```python
from build123d import *

# Parameters (mm, degrees)
SKETCH1_R                                         = 2.5
BOSS_EXTRUDE1_DEPTH                               = 5
SKETCH2_W                                         = 5
SKETCH2_H                                         = 55
BOSS_EXTRUDE2_DEPTH                               = 25
SKETCH3_W                                         = 72.3
SKETCH3_H                                         = 55
BOSS_EXTRUDE3_DEPTH                               = 5
BOSS_EXTRUDE4_DEPTH                               = 5
CUT_EXTRUDE1_REACH                                = 7
SKETCH5_R                                         = 2.5
CSK_FOR_M2_5_FLAT_HEAD_MACHINE_SCREW1_D           = 2.9
CSK_FOR_M2_5_FLAT_HEAD_MACHINE_SCREW1_CSINK_D     = 5.5
CSK_FOR_M2_5_FLAT_HEAD_MACHINE_SCREW1_CSINK_ANGLE = 90


with BuildPart() as part:
    # Sketch1 → Boss-Extrude1 (new body)
    with BuildSketch(Plane(origin=(0, 0, 0), x_dir=(0, 0, -1), z_dir=(1, 0, 0))):
        Polygon((-27.5, 17.5), (-17.5, 27.5), (17.5, 27.5), (27.5, 17.5), (27.5, -27.5), (-27.5, -27.5), align=None)
        Circle(SKETCH1_R, mode=Mode.SUBTRACT)
    extrude(amount=BOSS_EXTRUDE1_DEPTH)

    # Sketch2 → Boss-Extrude2 (add)
    with BuildSketch(Plane.XZ.offset(27.5)):
        with Locations((2.5, 0)):
            Rectangle(SKETCH2_W, SKETCH2_H)
    extrude(amount=BOSS_EXTRUDE2_DEPTH)

    # Sketch3 → Boss-Extrude3 (add)
    with BuildSketch(Plane.XZ.offset(52.5)):
        with Locations((-36.15, 0)):
            Rectangle(SKETCH3_W, SKETCH3_H)
    extrude(amount=-BOSS_EXTRUDE3_DEPTH)

    # Sketch4 → Boss-Extrude4 (add)
    with BuildSketch(Plane.ZY.offset(72.3)):
        Polygon((-17.5, 27.5), (-27.5, 17.5), (-27.5, -47.5), (27.5, -47.5), (27.5, 17.5), (17.5, 27.5), align=None)
    extrude(amount=-BOSS_EXTRUDE4_DEPTH)

    # Sketch5 → Cut-Extrude1 (cut, up to next)
    with BuildSketch(Plane(origin=(-67.3, 0, 0), x_dir=(0, 0, -1), z_dir=(1, 0, 0)), mode=Mode.PRIVATE) as cut_extrude1_sk1:
        Circle(SKETCH5_R)
    cut_extrude1_tool1 = extrude(cut_extrude1_sk1.sketch, amount=-CUT_EXTRUDE1_REACH, mode=Mode.PRIVATE) & part.part
    add(cut_extrude1_tool1.solids().sort_by_distance((-67.3, 0, 0))[0], mode=Mode.SUBTRACT)

    # CSK for M2.5 Flat Head Machine Screw1 (through all)
    with Locations(Plane(origin=(0, -47.5, 0), x_dir=(1, 0, 0), z_dir=(0, 1, 0))):
        with Locations((-16.15, 15), (-16.15, -15), (-46.15, -15), (-46.15, 15)):
            CounterSinkHole(CSK_FOR_M2_5_FLAT_HEAD_MACHINE_SCREW1_D / 2, CSK_FOR_M2_5_FLAT_HEAD_MACHINE_SCREW1_CSINK_D / 2, counter_sink_angle=CSK_FOR_M2_5_FLAT_HEAD_MACHINE_SCREW1_CSINK_ANGLE)


solid = part.part
```
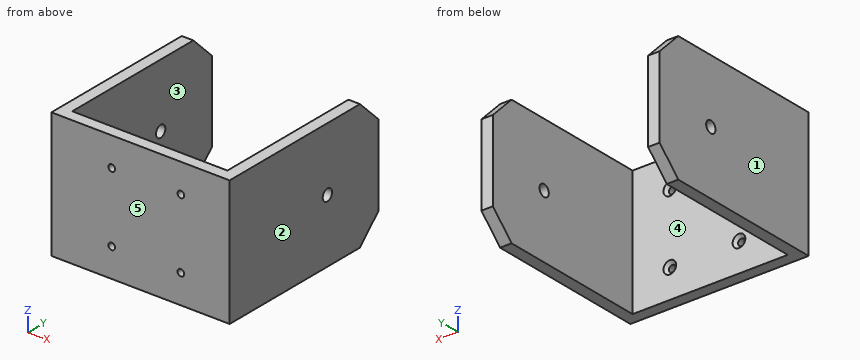
Input: part model. Units: mm. Frame: model coordinates. Face numbers are marked on the shaded views. A direction names the side the tool comes from. Coordinates: 2 decimals unless noted, no trailing zeros. Write each loop counter-clockwise with the first axis right and the second up, starting at its lowest first coordinate (ties: lowest second). Pieces come first, ordered by that corner, then holes. Notation, with made-up numbers: M -27.75,51.5 L -7.75,51.5 A26 cw -7.75,85.5 Z; hole C -1.5,32 d9. An arc over 180 degrees is marked long. Use one line per item in the form item = value.
Q1. Draft query along X for the marked faces 1, 2 and 3. Return one class per face: released by +X, released by -X, zero draft, split by the parting line, or undercut.
Answer below:
face_1 = released by -X
face_2 = released by +X
face_3 = undercut
Q2. Section D-D (y = -44). Return loops of the section in (x, z).
Answer below:
outline = M -72.3,-27.5 L -67.3,-27.5 L -67.3,27.5 L -72.3,27.5 Z; M 0,-27.5 L 5,-27.5 L 5,27.5 L 0,27.5 Z
Q3. Section B-B (y = 0). Return loops of the section in (x, z).
Answer below:
outline = M -72.3,-27.5 L -67.3,-27.5 L -67.3,-2.5 L -72.3,-2.5 Z; M -72.3,2.5 L -67.3,2.5 L -67.3,27.5 L -72.3,27.5 Z; M 0,-27.5 L 5,-27.5 L 5,-2.5 L 0,-2.5 Z; M 0,2.5 L 5,2.5 L 5,27.5 L 0,27.5 Z
Q4. Material intervals for probe 1 along X at (y, z) = (-50, -15); probe 2 along Z at (x, y) = (-46, -51); probe 3 along X at (y, z) = (10.5, 15), sorted ascending. Write a range as from..to.
Answer below:
probe_1 = -72.3..-47.6, -44.7..-17.6, -14.7..5
probe_2 = -27.5..-16.44, -13.56..13.56, 16.44..27.5
probe_3 = -72.3..-67.3, 0..5
Q5. Set-up query: the marked faces 4 and 5. Return all of +Z, -Z, +X, -X, +Y, -Y with unobstructed straight access to the full face (end or side cutting, diameter ignored); none if empty.
Answer below:
face_4 = +Z, -Z, +Y
face_5 = +Z, -Z, +X, -X, -Y
Q6. Section C-C (x = -16.15). Return loops of the section in (y, z), plus the area to 3 significant figures.
Answer below:
outline = M -52.5,-27.5 L -47.5,-27.5 L -47.5,-17.75 L -48.8,-16.45 L -52.5,-16.45 Z; M -52.5,-13.55 L -48.8,-13.55 L -47.5,-12.25 L -47.5,12.25 L -48.8,13.55 L -52.5,13.55 Z; M -52.5,16.45 L -48.8,16.45 L -47.5,17.75 L -47.5,27.5 L -52.5,27.5 Z
area = 243 mm²
Q7. Section A-A (z = 15). Return loops of the section in (x, y), plus the area to 3 significant figures.
Answer below:
outline = M -72.3,-52.5 L -47.6,-52.5 L -47.6,-48.8 L -48.9,-47.5 L -67.3,-47.5 L -67.3,27.5 L -72.3,27.5 Z; M -44.7,-52.5 L -17.6,-52.5 L -17.6,-48.8 L -18.9,-47.5 L -43.4,-47.5 L -44.7,-48.8 Z; M -14.7,-52.5 L 5,-52.5 L 5,27.5 L 0,27.5 L 0,-47.5 L -13.4,-47.5 L -14.7,-48.8 Z
area = 1,100 mm²
Q8. First-contact query: pin 1 (4.5 mm diameter, centred on x = -46.15, z = -15, fed in from +Y). Flat tip, straight axial feed; report the tip coordinate or a pass-through.
Answer below:
pin_1 = -48
